from build123d import *

# Parameters (mm, degrees)
SKETCH1_W                    = 184.15
SKETCH1_H                    = 152.4
SKETCH1_W_2                  = 133.35
SKETCH1_H_2                  = 101.6
BOSS_EXTRUDE1_DEPTH          = 1.5875
EDGE_FLANGE1_STRIP_W         = 26.35
EDGE_FLANGE1_STRIP_H         = 1.5875
EDGE_FLANGE1_STRIP_CUT_DEPTH = 152.4
EDGE_FLANGE1_DEPTH           = 152.4
EDGE_FLANGE2_STRIP_W         = 26.35
EDGE_FLANGE2_STRIP_H         = 1.5875
EDGE_FLANGE2_STRIP_CUT_DEPTH = 152.4
EDGE_FLANGE2_DEPTH           = 152.4
SKETCH16_W                   = 133.35
SKETCH16_H                   = 101.6
CUT_EXTRUDE1_DEPTH           = 1.5875
SKETCH17_W                   = 50.8
SKETCH17_H                   = 101.6
CUT_EXTRUDE2_DEPTH           = 1.5875
EDGE_FLANGE3_STRIP_W         = 26.35
EDGE_FLANGE3_STRIP_H         = 1.5875
EDGE_FLANGE3_STRIP_CUT_DEPTH = 152.4
EDGE_FLANGE3_DEPTH           = 152.4
EDGE_FLANGE4_STRIP_W         = 26.35
EDGE_FLANGE4_STRIP_H         = 1.5875
EDGE_FLANGE4_STRIP_CUT_DEPTH = 152.4
EDGE_FLANGE4_DEPTH           = 152.4


# Sheet-metal steps are written as plain solids
with BuildPart() as part:
    # Sketch1 → Boss-Extrude1 (new body)
    with BuildSketch(Plane.XY):
        with Locations((-92.075, 76.2)):
            Rectangle(SKETCH1_W, SKETCH1_H)
        with Locations((-92.075, 76.2)):
            Rectangle(SKETCH1_W_2, SKETCH1_H_2, mode=Mode.SUBTRACT)
    extrude(amount=BOSS_EXTRUDE1_DEPTH)

    # Edge-Flange1 strip (across the edge) → Edge-Flange1 strip cut (cut)
    with BuildSketch(Plane(origin=(0, 152.4, 0), x_dir=(-1, 0, 0), z_dir=(0, -1, 0))):
        with Locations((-1.5875, -0.79375)):
            Rectangle(EDGE_FLANGE1_STRIP_W, EDGE_FLANGE1_STRIP_H)
    extrude(amount=EDGE_FLANGE1_STRIP_CUT_DEPTH, mode=Mode.SUBTRACT)

    # Edge-Flange1 section (across the edge) → Edge-Flange1 (add)
    with BuildSketch(Plane(origin=(0, 152.4, 0), x_dir=(-1, 0, 0), z_dir=(0, -1, 0))):
        with BuildLine():
            Line((0, 10), (0, 100.0125))
            Line((0, 100.0125), (1.5875, 100.0125))
            Line((1.5875, 100.0125), (1.5875, 10))
            ThreePointArc((1.5875, 10), (4.516432188, 2.928932188), (11.5875, 0))
            Line((11.5875, 0), (11.5875, -1.5875))
            ThreePointArc((11.5875, -1.5875), (3.393900173, 1.806400173), (0, 10))
        make_face()
    extrude(amount=EDGE_FLANGE1_DEPTH)

    # Edge-Flange2 strip (across the edge) → Edge-Flange2 strip cut (cut)
    with BuildSketch(Plane(origin=(-1.5875, 152.4, -100.0125), x_dir=(0, 0, 1), z_dir=(0, -1, 0))):
        with Locations((-1.5875, -0.79375)):
            Rectangle(EDGE_FLANGE2_STRIP_W, EDGE_FLANGE2_STRIP_H)
    extrude(amount=EDGE_FLANGE2_STRIP_CUT_DEPTH, mode=Mode.SUBTRACT)

    # Edge-Flange2 section (across the edge) → Edge-Flange2 (add)
    with BuildSketch(Plane(origin=(-1.5875, 152.4, -100.0125), x_dir=(0, 0, 1), z_dir=(0, -1, 0))):
        with BuildLine():
            Line((0, 10), (0, 182.5625))
            Line((0, 182.5625), (1.5875, 182.5625))
            Line((1.5875, 182.5625), (1.5875, 10))
            ThreePointArc((1.5875, 10), (4.516432188, 2.928932188), (11.5875, 0))
            Line((11.5875, 0), (11.5875, -1.5875))
            ThreePointArc((11.5875, -1.5875), (3.393900173, 1.806400173), (0, 10))
        make_face()
    extrude(amount=EDGE_FLANGE2_DEPTH)

    # Sketch16 → Cut-Extrude1 (cut)
    with BuildSketch(Plane(origin=(0, 0, -100.0125), x_dir=(-1, 0, 0), z_dir=(0, 0, -1))):
        with Locations((92.075, 76.2)):
            Rectangle(SKETCH16_W, SKETCH16_H)
    extrude(amount=-CUT_EXTRUDE1_DEPTH, mode=Mode.SUBTRACT)

    # Sketch17 → Cut-Extrude2 (cut)
    with BuildSketch(Plane.ZY.offset(1.5875)):
        with Locations((-49.2125, 76.2)):
            Rectangle(SKETCH17_W, SKETCH17_H)
    extrude(amount=-CUT_EXTRUDE2_DEPTH, mode=Mode.SUBTRACT)

    # Edge-Flange3 strip (across the edge) → Edge-Flange3 strip cut (cut)
    with BuildSketch(Plane(origin=(-184.15, 152.4, -98.425), x_dir=(1, 0, 0), z_dir=(0, -1, 0))):
        with Locations((-1.5875, -0.79375)):
            Rectangle(EDGE_FLANGE3_STRIP_W, EDGE_FLANGE3_STRIP_H)
    extrude(amount=EDGE_FLANGE3_STRIP_CUT_DEPTH, mode=Mode.SUBTRACT)

    # Edge-Flange3 section (across the edge) → Edge-Flange3 (add)
    with BuildSketch(Plane(origin=(-184.15, 152.4, -98.425), x_dir=(1, 0, 0), z_dir=(0, -1, 0))):
        with BuildLine():
            Line((0, 10), (0, 23.8125))
            Line((0, 23.8125), (1.5875, 23.8125))
            Line((1.5875, 23.8125), (1.5875, 10))
            ThreePointArc((1.5875, 10), (4.516432188, 2.928932188), (11.5875, 0))
            Line((11.5875, 0), (11.5875, -1.5875))
            ThreePointArc((11.5875, -1.5875), (3.393900173, 1.806400173), (0, 10))
        make_face()
    extrude(amount=EDGE_FLANGE3_DEPTH)

    # Edge-Flange4 strip (across the edge) → Edge-Flange4 strip cut (cut)
    with BuildSketch(Plane(origin=(-184.15, 0, 0), x_dir=(1, 0, 0), z_dir=(0, 1, 0))):
        with Locations((-1.5875, -0.79375)):
            Rectangle(EDGE_FLANGE4_STRIP_W, EDGE_FLANGE4_STRIP_H)
    extrude(amount=EDGE_FLANGE4_STRIP_CUT_DEPTH, mode=Mode.SUBTRACT)

    # Edge-Flange4 section (across the edge) → Edge-Flange4 (add)
    with BuildSketch(Plane(origin=(-184.15, 0, 0), x_dir=(1, 0, 0), z_dir=(0, 1, 0))):
        with BuildLine():
            Line((0, 10), (0, 23.8125))
            Line((0, 23.8125), (1.5875, 23.8125))
            Line((1.5875, 23.8125), (1.5875, 10))
            ThreePointArc((1.5875, 10), (4.516432188, 2.928932188), (11.5875, 0))
            Line((11.5875, 0), (11.5875, -1.5875))
            ThreePointArc((11.5875, -1.5875), (3.393900173, 1.806400173), (0, 10))
        make_face()
    extrude(amount=EDGE_FLANGE4_DEPTH)


solid = part.part
Verification items for the finished model (mm, model axes). A direction names the side the tool comes from. Coordinates: 2 decimals unless noted, no trailing zeros. Order: outer loops, then holes, each group sorted by start corner. A loop starts at its lowest first (then second) coordinate and runs counter-clockwise, first axis right, second up.
Item 1: Depth check by flat-ended pin: pin 1 (0.5 mm diameter, centred on y = 81.5, z = 1, fed in from +X); pin 2 (1.7 mm diameter, centred on y = 52.5, z = -99, fed in from +X); pin 3 (0.5 mm diameter, centred on x = -1, y = 53.5, fed in from -Z). Enter the tip coordinate at first touch or a pass-through.
Filled in:
pin 1: stops at x = -7.26
pin 2: stops at x = -5.29
pin 3: stops at z = -93.66
Item 2: Section check D-D, the plane x = -163.5. Enter the section's corners in (y, z) (1 decimal), then the cut area to 3 significant figures.
Filled in:
outline: (0, -100) - (152.4, -100) - (152.4, -98.4) - (0, -98.4) - close; (0, 0) - (152.4, 0) - (152.4, 1.6) - (0, 1.6) - close
area: 484 mm2
Item 3: Section check C-C, the plane y = 124. Give the number of separate pieces and of enclosed holes in the cut face, then the cut area to 3 significant figures.
Filled in:
separate pieces: 4
enclosed holes: 0
area: 283 mm2
Item 4: Material ranges on L1, parallel to X at y = 22, z = -83; L2, parallel to Z at x = -106.5, y = 146 (1 decimal); L3, parallel to X at y = 26.5, z = -8, recorded low to high.
Filled in:
L1: x = -184.15 to -182.56, -1.59 to 0
L2: z = -100 to -98.4, 0 to 1.6
L3: x = -183.98 to -182.36, -1.79 to -0.17
Item 5: Section check B-B, the plane x = -96.5. Enter the section's corners in (y, z) (1 decimal).
Filled in:
outline: (0, -100) - (25.4, -100) - (25.4, -98.4) - (0, -98.4) - close; (0, 0) - (25.4, 0) - (25.4, 1.6) - (0, 1.6) - close; (127, -100) - (152.4, -100) - (152.4, -98.4) - (127, -98.4) - close; (127, 0) - (152.4, 0) - (152.4, 1.6) - (127, 1.6) - close
Item 6: Section check A-A, the plane z = -35.5. Enter the section's corners in (x, y).
Filled in:
outline: (-1.59, 0) - (0, 0) - (0, 25.4) - (-1.59, 25.4) - close; (-1.59, 127) - (0, 127) - (0, 152.4) - (-1.59, 152.4) - close
Item 7: Release check for a two-part mould opening along X. For faces 3 (the face through (-180.67, 75.13, -1.72)), 4 (the face through (0, 77, -75)), 5 (the face through (-93, 128, 0)), 6 (the face through (-182.562, 77, -81)) record: +X half, -X half, draft (parallel to the pull), parting line (faces both ways), or undercut.
Filled in:
face 3: -X half
face 4: +X half
face 5: undercut
face 6: undercut
Item 8: Access from +Z, -Z, +X, -X, +Y, -Y to the whole of each face (thin tool, end or side, straight path). Record for faces 1 (the face through (-4.59, 77.27, -95.57)), 2 (the face through (-3.304, 77.267, -96.528)).
Filled in:
face 1: +Y, -Y
face 2: -Z, +X, +Y, -Y
